Autodesk Inventor part; units mm, degrees
ref_plane "YZ Plane" through (0, 0, 0) normal (1, 0, 0) x (0, 1, 0)
ref_plane "XZ Plane" through (0, 0, 0) normal (0, 1, 0) x (-1, 0, 0)
ref_plane "XY Plane" through (0, 0, 0) normal (0, 0, 1) x (1, 0, 0)
sketch "Sketch1" plane through (0, 0, 0) normal (0, 0, 1) x (1, 0, 0)
  line L0 (0, 0) -> (247.65, 0)
  line L1 (247.65, 0) -> (247.65, 38.1)
  line L2 (247.65, 38.1) -> (0, 38.1)
  line L3 (0, 38.1) -> (0, 0)
  line L4 (286.1616, 0) -> (255.1962, 0)
  line L5 (255.1962, 0) -> (255.1962, 12.7)
  line L6 (255.1962, 12.7) -> (286.1616, 12.7)
  line L7 (286.1616, 12.7) -> (286.1616, 0)
  line L8 (247.65, 12.7) -> (200.66, 12.7)
  circle A0 centre (200.6294, 0) radius 47.0206
  line L9 (16.2468, 38.1) -> (16.2468, 12.7)
  line L10 (16.2468, 12.7) -> (155.3565, 12.7)
  line L11 (0, 12.7) -> (17.7951, 12.7)
  line L12 (179.5891, -42.0504) -> (75.8552, 12.7)
  point P0 (99.9175, 0)
  dimension "d0" = 247.65
  dimension "d1" = 38.1
  dimension "d2" = 12.7
  dimension "d3" = 30.9654
  dimension "d4" = 46.99
  dimension "d10" = 25.4
extrude "Extrusion1" add sketch "Sketch1" along normal blind 1.5875 contours L3 L11 L10 L12 L0 | L12 L10 A0 L0 | L0 A0 L12 | L3 L2 L9 L11 | A0 L2 L0 | L0 A0 L12 | L10 L9 L2 A0 | A0 L8 L1 | L8 A0 L2 L1
fillet "Fillet1" radius 28.575 1 edges at (247.65, 38.1, 0.7937)
fillet "Fillet2" radius 3.175 1 edges at (0, 38.1, 0.7937)
fillet "Fillet4" radius 3.175 1 edges at (0, 0, 0.7937)
fillet "Fillet5" radius 5.08 1 edges at (99.9175, 0, 0.7937)
sketch "Sketch3" plane through (0, 0, 1.5875) normal (0, 0, 1) x (1, 0, 0)
  line L0 (9.1438, 0) -> (9.1438, 11.176)
  line L1 (9.1438, 11.176) -> (-0.0002, 11.176)
  circle A0 centre (9.1438, 11.176) radius 2.54
  line L2 (9.1438, 11.176) -> (9.1438, 23.876)
  circle A1 centre (9.1438, 23.876) radius 2.54
  line L3 (9.1438, 17.526) -> (15.4938, 17.526)
  circle A2 centre (15.4938, 17.526) radius 2.54
  line L4 (15.4938, 17.526) -> (91.6938, 17.526)
  circle A3 centre (91.6938, 17.526) radius 2.54
  line L5 (91.6938, 17.526) -> (104.3938, 17.526)
  circle A4 centre (104.3938, 17.526) radius 2.54
  line L6 (104.3938, 17.526) -> (117.0938, 17.526)
  circle A5 centre (117.0938, 17.526) radius 4.445
  line L7 (9.1438, 11.176) -> (212.3438, 11.176)
  line L8 (9.1438, 23.876) -> (212.3438, 23.876)
  circle A6 centre (212.3438, 23.876) radius 2.54
  circle A7 centre (212.3438, 11.176) radius 2.54
  line L9 (125.3488, -8.3154) -> (158.5861, -26.9405)
  line L10 (158.5861, -26.9405) -> (180.7442, -39.3573)
  circle A8 centre (29.3464, 30.4847) radius 2.54
  circle A9 centre (84.6567, 30.4847) radius 2.54
  circle A10 centre (140.3584, 30.4847) radius 2.54
  circle A11 centre (192.9921, 30.4847) radius 2.54
  arc A12 (101.0303, -0.5874) -> (98.6591, 0) centre (98.6591, -5.08) ccw
  line L11 (98.6591, 0) -> (199.6241, 0)
  line L12 (199.6241, 0) -> (199.6241, -1.778)
  circle A13 centre (199.6241, -1.778) radius 4.445
  line L13 (219.075, 38.1) -> (3.175, 38.1)
  line L14 (140.3584, 38.1) -> (140.3584, 30.4847)
  line L15 (192.9921, 38.1) -> (192.9921, 30.4847)
  line L16 (84.6567, 38.1) -> (84.6567, 30.4847)
  line L17 (29.3464, 38.1) -> (29.3464, 30.4847)
  line L18 (221.0918, 31.9182) -> (221.0918, 30.4847)
  circle A14 centre (221.0918, 30.4847) radius 2.54
  line L19 (158.5861, -26.9405) -> (158.5861, -24.4005)
  circle A15 centre (158.5861, -24.4005) radius 2.54
  arc A16 (156.3864, -25.6705) -> (156.3703, -25.6989) centre (158.5861, -26.9405) ccw
  line L20 (180.7442, -39.3573) -> (180.7442, -34.2773)
  circle A17 centre (180.7442, -34.2773) radius 2.54
  line L21 (199.6056, -43.6188) -> (199.6056, -38.5388)
  circle A18 centre (199.6056, -38.5388) radius 2.54
  line L22 (223.6318, -36.189) -> (221.9594, -34.2773)
  circle A19 centre (221.9594, -34.2773) radius 2.54
  line L23 (235.2038, -25.0926) -> (233.5314, -23.1809)
  circle A20 centre (233.5314, -23.1809) radius 2.54
  line L24 (243.4585, 0) -> (240.9185, 0)
  circle A21 centre (240.9185, 0) radius 2.54
  line L25 (125.3488, -8.3154) -> (126.7888, -6.223)
  circle A22 centre (126.7888, -6.223) radius 2.54
  line L26 (49.7674, 4.225) -> (49.7674, 6.765)
  circle A23 centre (49.7674, 6.765) radius 2.54
  point P0 (0, 0)
  point P1 (94.2338, 17.526)
  point P2 (89.1538, 17.526)
  point P3 (6.6038, 11.176)
  point P4 (9.1438, 8.636)
  point P5 (18.0338, 17.526)
  point P6 (12.9538, 17.526)
  point P7 (11.6838, 23.876)
  point P8 (9.1438, 21.336)
  point P9 (125.756, -8.5435)
  dimension "d53" = 5.08
  dimension "d14" = 11.176
  dimension "d15" = 9.144
  dimension "d16" = 5.08
  dimension "d17" = 12.7
  dimension "d18" = 5.08
  dimension "d19" = 6.35
  dimension "d20" = 5.08
  dimension "d21" = 76.2
  dimension "d22" = 5.08
  dimension "d23" = 12.7
  dimension "d24" = 5.08
  dimension "d25" = 12.7
  dimension "d26" = 8.89
  dimension "d27" = 203.2
  dimension "d28" = 203.2
  dimension "d29" = 5.08
  dimension "d30" = 5.08
  dimension "d32" = 38.1
  dimension "d34" = 25.4
  dimension "d40" = 5.08
  dimension "d41" = 5.08
  dimension "d42" = 5.08
  dimension "d43" = 5.08
  dimension "d48" = 100.965
  dimension "d50" = 1.778
  dimension "d51" = 8.89
  dimension "d52" = 5.08
  dimension "d54" = 5.08
  dimension "d55" = 5.08
  dimension "d56" = 5.08
  dimension "d57" = 5.08
  dimension "d58" = 5.08
  dimension "d59" = 5.08
  dimension "d60" = 5.08
  dimension "d61" = 5.08
  dimension "d62" = 5.08
extrude "Extrusion2" cut sketch "Sketch3" against normal blind 25.4 contours A0 L1 L0 | A6 | A1 L8 L2 | L2 L8 A1 | A5 | A4 L6 L5 | L5 L6 A4 | A3 L5 L4 | L4 L5 A3 | A2 L4 L3 | L3 L4 A2 | A7 | L0 L7 A0 | L1 A0 L2 | L2 A0 L7 | A22 L9 | A17 | A15 L9 | L9 A15 | A8 | A11 | A10 | A9 | A13 | A14 | A18 | A19 | A20 | A21 | A23 picked at (125.3936, -5.8122)
properties part number "intake sled v5"
Here's how the part is built. I have some questions about the finished solid (model axes, mm). Round coordinates to 2 decimals unless told otherwise and drop trailing zeros. Order: outer loops, then holes, each group sorted by start corner. A loop starts at its lowest first (then second) coordinate and runs counter-clockwise, first axis right, second up. Notation, with made-up numbers: (-5.5, 49) -> (1.5, 49) arc R11 ccw to (1.5, 61) -> close; hole circle Ø11 at (-13.5, -0.75). An arc over 180 degrees is marked (long way). Return JSON: item names as keys, results as strings.
Q1. If we section it at B-B on x = 135: List the corners of the cut face in (y, z) for me, plus the area to 3 significant figures.
Filled sheet:
{"outline": "(-18.52, 0) -> (38.1, 0) -> (38.1, 1.59) -> (-18.52, 1.59) -> close", "area": "89.9 mm^2"}
Q2. If we mould it in two halves opening along X, with no side actions, what happens to faces 1 (the cylindrical face through (52.2, 7.5, 0.8)), 2 (the flat face through (140.86, -21.61, 0.78)), 3 (the flat face through (150, 6, 1.588))? For each: released by +X, released by -X, zero draft, split by the parting line, or undercut.
Filled sheet:
{"face 1": "undercut", "face 2": "released by -X", "face 3": "zero draft"}
Q3. If we section it at C-C on x = 165: List the corners of the cut face in (y, z) for me.
Filled sheet:
{"outline": "(-34.35, 0) -> (38.1, 0) -> (38.1, 1.59) -> (-34.35, 1.59) -> close"}
Q4. If we section it at A-A on z = 1.2: Give the number of separate pieces and of enclosed holes in the cut face, plus the area to 3 significant figures.
Filled sheet:
{"separate pieces": "1", "enclosed holes": "22", "area": "13,100 mm^2"}
Q5. I need wall thicknesses on line 1 along X through (y, z) = (11.5, 0.85); line 2 along Y through (x, z) = (159, 1.55); line 3 along X through (y, z) = (13.5, 0.75). Which ranges of each line are inside material? Lowest first, please. Write a range as from..to.
Filled sheet:
{"line 1": "x = 0..6.62, 11.66..209.82, 214.86..247.58", "line 2": "y = -31.18..-26.91, -21.89..38.1", "line 3": "x = 0..8.12, 10.17..115.21, 118.98..211.32, 213.37..247.37"}
Q6. For pin 1 Ø4.5 at (x, y) = (212.34, 11.18) entering from +Z, with a flat end and sliding along its axis, tell me the tip position at first contact or that it passes through.
Filled sheet:
{"pin 1": "passes through"}
